CAD build for the part. Positions are in the model's coordinates, mm. Face numbers are marked on the shaded views. A direction names the side the tool comes from. Round coordinates to 2 decimals unless told otherwise and drop trailing zeros. Loops run counter-clockwise (first coordinate to the right, second up) from the corner with the lowest first, then second, coordinate; pieces in that order, holes last. Notation, with made-up numbers: M 42.25,54 L 46.25,54 A25 ccw 46.25,84 Z; hole C 77.5,-19.75 d9. An arc over 180 degrees is marked long. Use a Markdown table: item, result. Add a question column.
(1) Wall check: L1, parallel to Y at x = -4, z = 5.75; L2, parallel to X at y = 23.5, z = 6 (3 decimals); L3, parallel to Y at x = -5.75, z = 3.81. Give the ranges that are in metal, low to high.
(2) Band-saw the part on C-C, the plane x = -17.5. Write the cut outline in (y, z), and give its area (3 significant figures).
(3) Flat gauge pins, fed straight in: P1, Ø2.5, axis at y = 23.5, z = 3.5, coming from the -X side; P2, Ø2, axis at y = 18, z = 4.5, coming from the +X side; P3, Ø3, axis at y = 29.64, z = 3.81, coming from the +X side; P4, Ø3, axis at y = -11, z = 6.5, coming from the +X side. Where does each tip first touch, or does it go through?
(4) Band-saw the part on B-B, the plane z = 5.5. Write the cut outline in (x, y) (3 decimals), and give its area (3 significant figures).
(5) Band-saw the part on D-D, the plane x = 0. Write the cut outline in (y, z).
(6) Band-saw the part on A-A, the plane y = 0. Write the cut outline in (x, z), and give its area (3 significant figures).
(7) Which spindle directions (+Z, -Z, +X, -X, +Y, -Y) get a long thin tool onto all of the face, cutting with end or side? Do the marked faces 1 and 2. Say none if no direction does.
(8) Two-plate mould, pull along Z, no slides. Class the marked faces 3, 4 and 5: released by +Z, released by -Z, zero draft, split by the parting line, or undercut.
from build123d import *

# Parameters (mm, degrees)
F1_DEPTH      = 7.62
F2_R          = 2.54
F3_DEPTH      = 25.4
F3_DEPTH_BACK = 25.4
F4_R          = 3.81
F5_R          = 3.80999


# Not quite as in the source:
# - a fillet or chamfer is up to 0.001 mm smaller than in the source, because OpenCascade refuses the exact size


with BuildPart() as f1:
    # F0 (on Top) → F1 (new body)
    with BuildSketch(Plane.XY):
        with BuildLine():
            ThreePointArc((3.175, 20.0704203992), (0, -20.32), (-3.175, 20.0704203992))
            Line((-3.175, 20.0704203992), (-3.175, 33.4507006653))
            Line((-3.175, 33.4507006653), (-6.985, 33.4507006653))
            Line((-6.985, 33.4507006653), (-20.4920611043, 15.0078456714))
            ThreePointArc((-20.4920611043, 15.0078456714), (0, -25.4), (20.4920611043, 15.0078456714))
            Line((20.4920611043, 15.0078456714), (6.985, 33.4507006653))
            Line((6.985, 33.4507006653), (3.175, 33.4507006653))
            Line((3.175, 33.4507006653), (3.175, 20.0704203992))
        make_face()
    extrude(amount=F1_DEPTH)

    # F2 (on face) → F3 (cut, two sides)
    with BuildSketch(Plane.YZ.offset(-3.175)) as f3_sk:
        with Locations((29.6407006653, 3.81)):
            Circle(F2_R)
    extrude(amount=F3_DEPTH, mode=Mode.SUBTRACT)
    extrude(f3_sk.sketch, amount=-F3_DEPTH_BACK, mode=Mode.SUBTRACT)

    # F4
    f4_edges = [f1.edges().sort_by_distance(p)[0] for p in [
        (-5.08, 33.450701, 0),
        (5.08, 33.450701, 0),
    ]]
    fillet(f4_edges, radius=F4_R)

    # F5 (radius 3.81 in the source; OpenCascade refuses exactly that, so slightly less here)
    f5_edges = [f1.edges().sort_by_distance(p)[0] for p in [
        (-5.08, 33.450701, 7.62),
        (5.08, 33.450701, 7.62),
    ]]
    fillet(f5_edges, radius=F5_R)


solid = f1.part
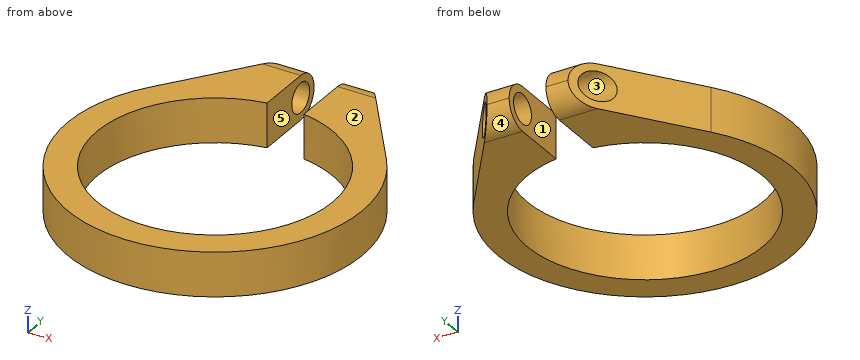
Return value:
| question | item | result |
|---|---|---|
| 1 | L1 | -25.08 to -19.92, 19.92 to 28, 31.28 to 32.92 |
| 1 | L2 | -14.273 to -3.175, 3.175 to 14.273 |
| 1 | L3 | -24.74 to -19.49, 19.49 to 27.1, 32.18 to 33.45 |
| 2 | outline | M -18.41,0 L -10.33,0 L -10.33,7.62 L -18.41,7.62 Z; M 10.33,0 L 19.09,0 L 19.09,7.62 L 10.33,7.62 Z |
| 2 | area | 128 mm^2 |
| 3 | P1 | x = -15.19 |
| 3 | P2 | x = 19.03 |
| 3 | P3 | through |
| 3 | P4 | x = 23.56 |
| 4 | outline | M -20.492,15.008 A25.4 ccw long 20.492,15.008 L 11.164,27.745 L 3.175,27.745 L 3.175,20.07 A20.32 cw long -3.175,20.07 L -3.175,27.745 L -11.164,27.745 Z; M -8.387,31.537 L -3.175,31.537 L -3.175,33.055 L -7.275,33.055 Z; M 3.175,31.537 L 8.387,31.537 L 7.275,33.055 L 3.175,33.055 Z |
| 4 | area | 801 mm^2 |
| 5 | outline | M -25.4,0 L -20.32,0 L -20.32,7.62 L -25.4,7.62 Z |
| 6 | outline | M -25.4,0 L -20.32,0 L -20.32,7.62 L -25.4,7.62 Z; M 20.32,0 L 25.4,0 L 25.4,7.62 L 20.32,7.62 Z |
| 6 | area | 77.4 mm^2 |
| 7 | face 1 | +Z, -Z, +Y |
| 7 | face 2 | +Z, +X, -X, +Y, -Y |
| 8 | face 3 | undercut |
| 8 | face 4 | released by -Z |
| 8 | face 5 | zero draft |
